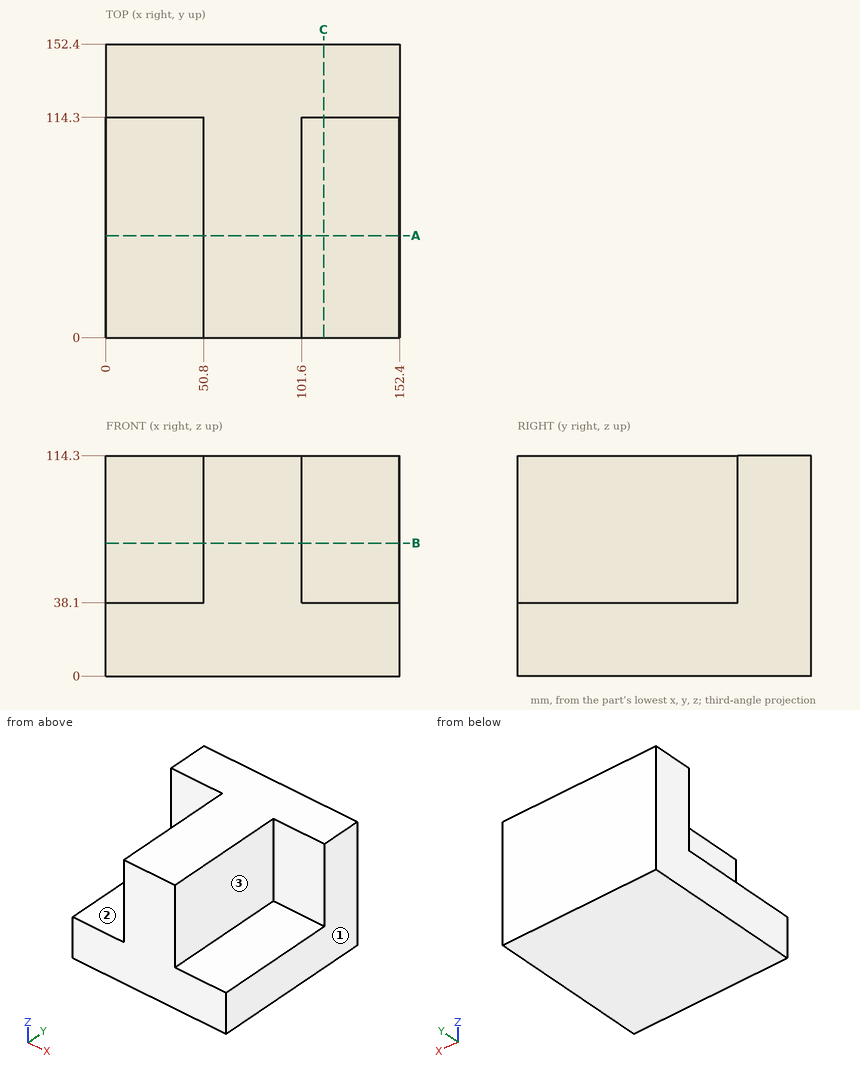
Check sheet for the drawn part. Datum: minimum x, y, z corner. Units: mm. A direction names the side the tool comes from. Coordinates: 2 decimals unless noted, no trailing zeros. Loops run counter-clockwise (first coordinate to the right, second up) from the corner with the lowest first, then second, coordinate; pieces in that order, holes last. Notation, with made-up numbers: (17.25, -15.5) - (41.25, -15.5) arc R31 ccw to (41.25, 9.5) - close; hole circle Ø9 at (38, 0). An arc over 180 degrees is marked (long way). Put each result on its own line as item: value.
Item 1: Section check B-B (z = 69). Enter the section's corners in (x, y).
Conclusion:
outline: (0, 114.3) - (50.8, 114.3) - (50.8, 0) - (101.6, 0) - (101.6, 114.3) - (152.4, 114.3) - (152.4, 152.4) - (0, 152.4) - close
Item 2: Gauge pin test, flat ends, axial feed: pin 1 Ø15 at (x, z) = (18, 64) entering from -Y; pin 2 Ø1 at (y, z) = (62.5, 92) entering from +X; pin 3 Ø23 at (y, z) = (84.5, 79) entering from -X. Record the tip position at first contact, or that the pin passes through.
Conclusion:
pin 1: stops at y = 114.3
pin 2: stops at x = 101.6
pin 3: stops at x = 50.8
Item 3: Scan lines: line 1 along Z through (x, y) = (16, 23); line 2 along Y through (x, z) = (134.5, 44); line 3 along X through (y, z) = (85.5, 89.5). Record each from-to range of solid material in increasing order.
Conclusion:
line 1: z = 0 to 38.1
line 2: y = 114.3 to 152.4
line 3: x = 50.8 to 101.6
Item 4: Section check A-A (y = 53). Enter the section's corners in (x, z), then the cut area to 3 significant figures.
Conclusion:
outline: (0, 0) - (152.4, 0) - (152.4, 38.1) - (101.6, 38.1) - (101.6, 114.3) - (50.8, 114.3) - (50.8, 38.1) - (0, 38.1) - close
area: 9,680 mm2
Item 5: Set-up check for the marked faces 1, 2 and 3: record each of +Z, -Z, +X, -X, +Y, -Y from which the full face is reachable in a straight line by a thin tool's end or side.
Conclusion:
face 1: +Z, -Z, +X, +Y, -Y
face 2: +Z, -X, -Y
face 3: +Z, +X, -Y
Item 6: Section check C-C (x = 113). Enter the section's corners in (y, z).
Conclusion:
outline: (0, 0) - (152.4, 0) - (152.4, 114.3) - (114.3, 114.3) - (114.3, 38.1) - (0, 38.1) - close
